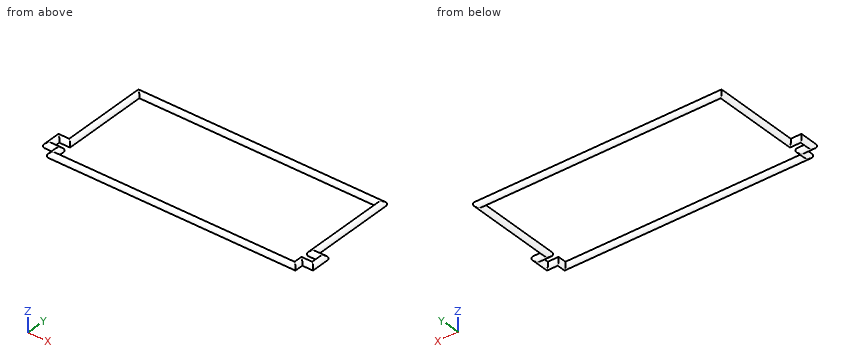
from build123d import *

# Parameters (mm, degrees)
SKETCH2_R = 0.7


with BuildPart() as part:
    # Sweep1: sweep along a path in Sketch1
    with BuildLine(Plane.XY) as sweep1_path:
        Line((0, 25.2), (56.5, 25.2))
        Line((56.5, 25.2), (56.5, 5.05))
        Line((56.5, 5.05), (59, 5.05))
        Line((59, 5.05), (59, 2))
        Line((59, 2), (56.5, 2))
        Line((56.5, 2), (56.5, 0))
        Line((56.5, 0), (0, 0))
        Line((0, 0), (0, 2))
        Line((0, 2), (-2.5, 2))
        Line((-2.5, 2), (-2.5, 5.05))
        Line((-2.5, 5.05), (0, 5.05))
        Line((0, 5.05), (0, 25.2))
    # Sketch2 → Sweep1 (sweep)
    with BuildSketch(Plane(origin=(0, 0, 0), x_dir=(0, 0, -1), z_dir=(1, 0, 0))):
        Circle(SKETCH2_R)
    sweep(path=sweep1_path.line, transition=Transition.RIGHT)


solid = part.part
Design review of the part built by this model. Coordinates are the model's own, in mm. Give positions to 0.01 mm unless a question says otherwise; leave off trailing zeros. Loops run counter-clockwise (first coordinate to the right, second up) from the corner with the lowest first, then second, coordinate; pieces in that order, holes last. Notation, with made-up numbers: M 32.25,69 L 52.25,69 A11 ccw 52.25,89 Z; hole C -29,23.25 d5. An arc over 180 degrees is marked long. Answer as a JSON object with one key per item and string values.
Item 1: Wall thickness on line 1 along Y through (x, z) = (1.5, -0.1); line 2 along X through (y, z) = (15.5, 0.1); line 3 along X through (y, z) = (9.25, -0.35): over which ranges is each line inside the solid? List them lowest first.
Output values:
{"line 1": "y = -0.69 to 0.69, 24.51 to 25.89", "line 2": "x = -0.69 to 0.69, 55.81 to 57.19", "line 3": "x = -0.61 to 0.61, 55.89 to 57.11"}
Item 2: We need section C-C (z = -0.45). State the section outline as (x, y) points.
Output values:
{"outline": "M -3.04,1.46 L -0.54,1.46 L -0.54,-0.54 L 57.04,-0.54 L 57.04,1.46 L 59.54,1.46 L 59.54,5.59 L 57.04,5.59 L 57.04,25.74 L -0.54,25.74 L -0.54,5.59 L -3.04,5.59 Z; hole M -1.96,2.54 L 0.54,2.54 L 0.54,0.54 L 55.96,0.54 L 55.96,2.54 L 58.46,2.54 L 58.46,4.51 L 55.96,4.51 L 55.96,24.66 L 0.54,24.66 L 0.54,4.51 L -1.96,4.51 Z"}
Item 3: We need section D-D (y = 20). State the section outline as (x, z) points, and give its area (3 significant figures).
Output values:
{"outline": "C 0,0 d1.4; C 56.5,0 d1.4", "area": "3.08 mm2"}
Item 4: We need section A-A (x = 56.5). State the section outline as (y, z) points.
Output values:
{"outline": "M 0,-0.7 L 2,-0.7 A0.7 ccw 2,0.7 L 0,0.7 A0.7 ccw Z; M 5.05,-0.7 L 25.2,-0.7 A0.7 ccw 25.2,0.7 L 5.05,0.7 A0.7 ccw Z"}
Item 5: We need section B-B (y = 5.05). State the section outline as (x, z) points.
Output values:
{"outline": "M -2.5,-0.7 L 0,-0.7 A0.7 ccw 0,0.7 L -2.5,0.7 A0.7 ccw Z; M 56.5,-0.7 L 59,-0.7 A0.7 ccw 59,0.7 L 56.5,0.7 A0.7 ccw Z"}
